The model under review builds one solid part; all positions refer to its coordinate system, in mm. Give positions to 0.01 mm unless a question says otherwise; leave off trailing zeros. Loops run counter-clockwise (first coordinate to the right, second up) from the corner with the lowest first, then second, coordinate; pieces in that order, holes last. Notation, with made-up numbers: M -35,39 L 13,39 A14 ccw 13,53 Z; hole C 47,-31.75 d8. An arc over 180 degrees is marked long. One line per item, written item: value. Start each with the question number.
Q1. For pin 1 (1 mm diameter, centred on y = 2.5, z = 1, fed in from -X); pin 2 (3 mm diameter, centred on x = 0, z = 0.5, fed in from -Y); pin 3 (1 mm diameter, centred on x = -1, y = 2, fed in from +Z), all flat-tipped, find the tip position at first contact; note any pin that passes through.
Q2. We need section A-A on x = -1.2. Write out the cut boundary in (y, z).
Q3. To check wall thickness, follow line 1 along Z through (x, y) = (-2.15, 0.6); line 2 along Y through (x, z) = (-0.85, -0.7); line 3 along Z through (x, y) = (-1.45, 0.35). State the ranges of each line that lie inside material, in increasing order. Write a range as from..to.
Autodesk Inventor part; units mm, degrees
ref_plane "YZ Plane" through (0, 0, 0) normal (1, 0, 0) x (0, 1, 0)
ref_plane "XZ Plane" through (0, 0, 0) normal (0, 1, 0) x (-1, 0, 0)
ref_plane "XY Plane" through (0, 0, 0) normal (0, 0, 1) x (1, 0, 0)
sketch "Sketch1" plane through (0, 0, 0) normal (0, 1, 0) x (-1, 0, 0)
  line L0 (1.5, -1.6689) -> (-1.5, -1.6689)
  line L1 (-1.5, -3.6689) -> (1.5, -3.6689)
  arc A0 (2.5, -2.6689) -> (1.5, -1.6689) centre (1.5, -2.6689) ccw
  arc A1 (1.5, -3.6689) -> (2.5, -2.6689) centre (1.5, -2.6689) ccw
  arc A2 (-2.5, -2.6689) -> (-1.5, -3.6689) centre (-1.5, -2.6689) ccw
  arc A3 (-1.5, -1.6689) -> (-2.5, -2.6689) centre (-1.5, -2.6689) ccw
  line L2 (1.5, -2.6689) -> (-1.5, -2.6689) construction
  point P0 (2.5, -1.6689)
  point P1 (-2.5, -3.6689)
  point P2 (2.5, -3.6689)
  point P3 (-2.5, -2.6689)
  dimension "d1" = 5
  dimension "d2" = 2
  dimension "d3" = 1
  dimension "d4" = 1
sketch "Sketch2" plane through (0, 0, 0) normal (1, 0, 0) x (0, 1, 0)
  line L0 (0, -2.6689) -> (0, 1.3311) construction
  arc A0 (0, -2.6689) -> (0, 1.3311) centre (0, -0.6689) ccw
  point P0 (0, 0)
  dimension "d5" = 4
sweep "Sweep1" add profiles "Sketch1" path "Sketch2"
properties part number "seguro"
Solved:
1. pin 1: x = -2.36
1. pin 2: y = 0
1. pin 3: z = 1.93
2. outline: M 0,-3.67 A3 ccw 0,2.33 L 0,0.33 A1 cw 0,-1.67 Z
3. line 1: -3.36..-1.75, 0.42..2.03
3. line 2: 1..3
3. line 3: -3.65..-1.61, 0.27..2.31
